Autodesk Inventor part; units mm, degrees
ref_plane "Work Plane1" through (79.5, 0, 0) normal (1, 0, 0) x (0, 0, -1)
ref_plane "YZ Plane" through (0, 0, 0) normal (1, 0, 0) x (0, 1, 0)
ref_plane "XZ Plane" through (0, 0, 0) normal (0, 1, 0) x (-1, 0, 0)
sketch "Sketch1" plane through (0, 0, 0) normal (1, 0, 0) x (0, 1, 0)
  line L0 (0, 0) -> (0, -85)
  line L1 (0, 0) -> (39.6107, -5.5669)
  line L2 (0, 0) -> (40, 0) construction
  line L3 (39.6107, -5.5669) -> (66.6924, -41.5055)
  line L4 (66.6924, -41.5055) -> (49.9211, -54.1436)
  line L5 (49.9211, -54.1436) -> (47.2715, -49.9034)
  line L6 (0, -85) -> (4, -85)
  line L7 (5, -55) -> (4, -85)
  line L8 (5, -55) -> (47.2715, -49.9034)
  dimension "d0" = 85
  dimension "d1" = 40
  dimension "d2" = 8
  dimension "d3" = 45
  dimension "d4" = 135
  dimension "d5" = 21
  dimension "d6" = 5
  dimension "d7" = 85
  dimension "d12" = 4
  dimension "d13" = 5
  dimension "d50" = 30
extrude "Extrusion1" add sketch "Sketch1" along normal blind 3
sketch "Sketch2" plane through (3, 0, 0) normal (1, 0, 0) x (0, 0, -1)
  line L0 (0, 0) -> (85, 0)
  line L1 (85, 0) -> (85, 4)
  line L2 (85, 4) -> (55, 5)
  line L3 (49.9034, 47.2715) -> (54.1436, 49.9211)
  line L4 (54.1436, 49.9211) -> (41.5055, 66.6924)
  line L5 (41.5055, 66.6924) -> (5.5669, 39.6107)
  line L6 (5.5669, 39.6107) -> (0, 0)
  line L7 (49.9034, 47.2715) -> (54.1436, 49.9211)
  line L8 (51.1436, 48.0464) -> (40.9151, 62.491)
  line L9 (41.5055, 66.6924) -> (5.5669, 39.6107)
  line L10 (54.1436, 49.9211) -> (41.5055, 66.6924)
  line L11 (40.9151, 62.491) -> (8.3648, 37.9627)
  line L12 (8.3648, 37.9627) -> (3, 3)
  line L13 (5.5669, 39.6107) -> (0, 0)
  line L14 (3, 3) -> (85, 3)
  line L15 (85, 0) -> (85, 4)
  line L16 (85, 3) -> (85, 0)
  line L17 (0, 0) -> (85, 0)
  line L18 (85, 0) -> (0, 0)
  line L19 (0, 0) -> (5.5669, 39.6107)
  line L20 (5.5669, 39.6107) -> (41.5055, 66.6924)
  line L21 (41.5055, 66.6924) -> (54.1436, 49.9211)
  line L22 (54.1436, 49.9211) -> (51.1436, 48.0464)
  line L23 (55, 5) -> (49.9034, 47.2715)
  dimension "d14" = 3
  dimension "d15" = 3
  dimension "d16" = 3
  dimension "d17" = 3
  dimension "d18" = 3
  dimension "d21" = 3
  dimension "d22" = 3
  dimension "d23" = 3
extrude "Extrusion2" add sketch "Sketch2" along normal blind 153 contours L6 L5 L4 L3 L8 L11 L12 L14 L1 L0
ref_plane "Work Plane1" through (79.5, 0, 0) normal (1, 0, 0) x (0, 0, -1)
mirror "Mirror1" about plane through (79.5, 0, 0) normal (1, 0, 0) of "Extrusion1"
sketch "Sketch3" plane through (159, 0, -85) normal (1, 0, 0) x (0, 0, -1)
  line L0 (-85, 0) -> (0, 0)
  line L1 (-79.4331, 39.6107) -> (-85, 0)
  circle A0 centre (-62.193, 25.4) radius 1.5
  circle A1 centre (-49.984, 30) radius 1.5
  dimension "d28" = 25.4
  dimension "d29" = 30
  dimension "d31" = 19.05
  dimension "d32" = 30.5
  dimension "d33" = 3
  dimension "d34" = 3
extrude "Extrusion3" cut sketch "Sketch3" against normal blind 200
sketch "Sketch4" plane through (0, 0, 0) normal (0, 0.1392, 0.9903) x (1, 0, 0)
  line L0 (0, 0) -> (159, 0)
  line L1 (0, 40) -> (0, 0)
  line L2 (159, 40) -> (159, 0)
  circle A0 centre (25.4, 31.75) radius 1.5
  circle A1 centre (25.4, 11.1125) radius 1.5
  circle A2 centre (133.6, 31.75) radius 1.5
  circle A3 centre (133.6, 11.1125) radius 1.5
  dimension "d37" = 11.1125
  dimension "d38" = 31.75
  dimension "d39" = 25.4
  dimension "d40" = 31.75
  dimension "d41" = 11.1125
  dimension "d42" = 25.4
  dimension "d43" = 3
  dimension "d44" = 3
  dimension "d45" = 3
  dimension "d46" = 3
extrude "Extrusion4" cut sketch "Sketch4" against normal blind 10
properties part number "plowV4"
Input: part model. Units: mm. Frame: model coordinates. A direction names the side the tool comes from. Give positions to 0.01 mm unless a question says otherwise; leave off trailing zeros. Loops run counter-clockwise (first coordinate to the right, second up) from the corner with the lowest first, then second, coordinate; pieces in that order, holes last.
1) Mould query, pull axis Y, two halves, no side actions, for faces 1 (the flat face through (80.61, 49.17, -52.94)), 2 (the flat face through (81, 0, -43)), 3 (the flat face through (0, 25, -32)). Classes: released by +Y, released by -Y, zero draft, split by the parting line, or undercut.
A:
face 1: undercut
face 2: released by -Y
face 3: zero draft
2) Section query A-A on x = 109.5. Return the cut outline in (y, z).
A:
outline: (0, -85) - (3, -85) - (3, -3) - (37.96, -8.36) - (62.49, -40.92) - (48.05, -51.14) - (49.92, -54.14) - (66.69, -41.51) - (39.61, -5.57) - (0, 0) - close
3) Line query: L1, parallel to X at y = 30.5, z = -31; L2, parallel to Y at x = 21, z = -65; L3, parallel to Z at x = 81, y = 53.5. Output: solid intervals per line, ascending.
A:
L1: x = 0 to 3, 156 to 159
L2: y = 0 to 3
L3: z = -51.45 to -47.28, -28.98 to -24
4) Contact query for flat-ended pins moving along their axis: pin 1 (18 mm diameter, centred on y = 28.5, z = -43, fed in from -X); pin 2 (1 mm diameter, centred on x = 44, z = -23.5, fed in from +Y); pin 3 (3 mm diameter, centred on x = 31.5, z = -20, fed in from +Y); pin 4 (24.5 mm diameter, centred on x = 103.5, z = -54, fed in from +Y). Output: stop coordinate, or through.
A:
pin 1: stops at x = 0
pin 2: stops at y = 53.5
pin 3: stops at y = 51.62
pin 4: stops at y = 66.37
5) Reachability of faces 4 (the flat face through (78.43, 20.73, -5.72)), 5 (the cylindrical face through (1.521, 23.936, -22.482)), 6 (the flat face through (157.521, 26.432, -52.416)), 7 (the flat face through (80.613, 53.341, -23.788)), 8 (the flat face through (78.43, 50.4, -24.87)) from +Z, -Z, +X, -X, +Y, -Y: full face, straight path, thin tool, end or side. Return the list, or none.
A:
face 4: -Z
face 5: +X, -X
face 6: -Z, +X, -X
face 7: +Z, +X, -X, +Y
face 8: none
